Part model, mm, in its own coordinate system. Give positions to 0.01 mm unless a question says otherwise; leave off trailing zeros. Loops run counter-clockwise (first coordinate to the right, second up) from the corner with the lowest first, then second, coordinate; pieces in that order, holes last. Notation, with made-up numbers: (88, 12.25) -> (123, 12.25) arc R12 ccw to (123, 25.25) -> close; hole circle Ø9 at (70, -3.75). An arc over 180 degrees is marked (long way). One line per question, with ' | ' between items.
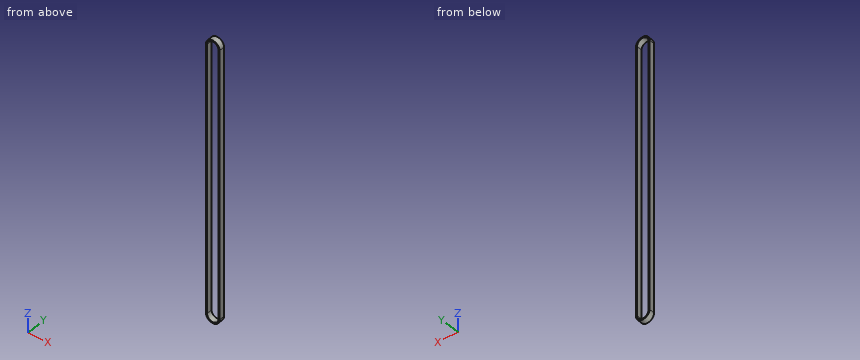
Autodesk Inventor part; units mm, degrees
ref_plane "YZ Plane" through (0, 0, 0) normal (1, 0, 0) x (0, 1, 0)
ref_plane "XZ Plane" through (0, 0, 0) normal (0, 1, 0) x (-1, 0, 0)
ref_plane "XY Plane" through (0, 0, 0) normal (0, 0, 1) x (1, 0, 0)
sketch "Sketch1" plane through (0, 0, 0) normal (0, 1, 0) x (-1, 0, 0)
  line L0 (0, 375) -> (0, -375) construction
  line L1 (15, 360) -> (15, -360)
  line L2 (-15, -360) -> (-15, 360)
  arc A0 (15, 360) -> (-15, 360) centre (0, 360) ccw
  arc A1 (-15, -360) -> (15, -360) centre (0, -360) ccw
  line L3 (18, -360) -> (18, 360)
  arc A2 (18, 360) -> (-18, 360) centre (0, 360) ccw
  line L4 (-18, 360) -> (-18, -360)
  arc A3 (-18, -360) -> (18, -360) centre (0, -360) ccw
  point P0 (0, 0)
  point P1 (0, 0)
  dimension "d0" = 15
  dimension "d1" = 720
  dimension "d2" = 3
extrude "Extrusion1" add sketch "Sketch1" along normal blind 15
properties part number "X_Zahnriemen"
1) Saw through at A-A (z = -198). Give the cut face in (x, y), and give its area (3 significant figures).
Found:
outline: (-18, 0) -> (-15, 0) -> (-15, 15) -> (-18, 15) -> close; (15, 0) -> (18, 0) -> (18, 15) -> (15, 15) -> close | area: 90.0 mm2
2) Saw through at B-B (x = 0). Give the cut face in (y, z), and give its area (3 significant figures).
Found:
outline: (0, -378) -> (15, -378) -> (15, -375) -> (0, -375) -> close; (0, 375) -> (15, 375) -> (15, 378) -> (0, 378) -> close | area: 90.0 mm2
3) Pin check, flat tips, straight feed: P1, Ø6, axis at x = -2, y = 6.5, coming from the +Z side; P2, Ø1, axis at x = -13, y = 13, coming from the -Z side; P3, Ø3, axis at x = -10, y = 12.5, coming from the -Z side. Stop position of each tip, or through.
Found:
P1: z = 378 | P2: z = -372.95 | P3: z = -375.87
4) Drill centre lines: line 1 (X direction, y = 5.75, z = 233.5); line 2 (Z direction, x = -1.5, y = 10.5); line 3 (Z direction, x = 0, y = 4.5). Where is each one in solid material? Low to high.
Found:
line 1: -18 to -15, 15 to 18 | line 2: -377.94 to -374.92, 374.92 to 377.94 | line 3: -378 to -375, 375 to 378
5) Saw through at C-C (y = 9). Give the cut face in (x, z).
Found:
outline: (-18, -360) arc R18 ccw to (18, -360) -> (18, 360) arc R18 ccw to (-18, 360) -> close; hole (-15, -360) arc R15 ccw to (15, -360) -> (15, 360) arc R15 ccw to (-15, 360) -> close
